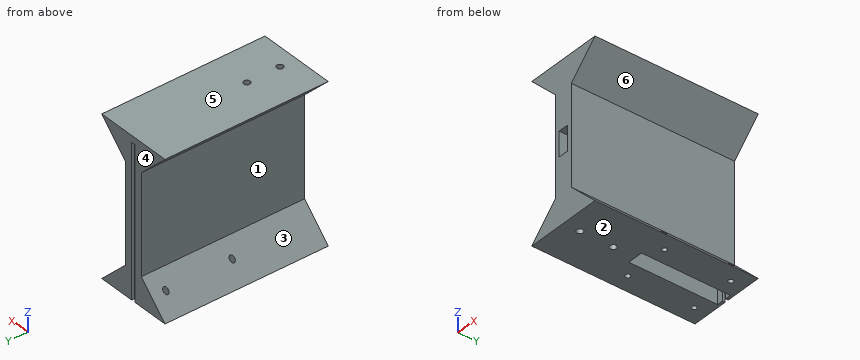
from build123d import *

# Parameters (mm, degrees)
BOSS_EXTRUDE1_DEPTH            = 125
SKETCH3_W                      = 12
SKETCH3_H                      = 68
CUT_EXTRUDE1_DEPTH             = 115.57
SKETCH4_W                      = 3.175
SKETCH4_H                      = 115.57
CUT_EXTRUDE2_DEPTH             = 3
CUT_EXTRUDE3_REACH             = 143.943
SKETCH5_W                      = 8
SKETCH5_H                      = 19.05
SKETCH6_R                      = 2.45745
CUT_EXTRUDE4_DEPTH             = 25.4
CUT_EXTRUDE5_START             = -25.4
SKETCH7_R                      = 2.45745
CUT_EXTRUDE5_DEPTH             = 25.4
TAP_DRILL_FOR_10_24_TAP1_D     = 3.7973
TAP_DRILL_FOR_10_24_TAP1_DEPTH = 30
TAP_DRILL_FOR_10_24_TAP1_TIP   = 1.140824014


with BuildPart() as part:
    # Sketch1 → Boss-Extrude1 (new body)
    with BuildSketch(Plane(origin=(0, 0, 0), x_dir=(1, 0, 0), z_dir=(0, 1, 0))):
        Polygon((-29.725, -60.325), (29.725, -60.325), (7.5, -38.1), (7.5, 38.1), (29.725, 60.325), (-29.725, 60.325), (-7.5, 38.1), (-7.5, -38.1), align=None)
    extrude(amount=BOSS_EXTRUDE1_DEPTH)

    # Sketch3 → Cut-Extrude1 (cut)
    with BuildSketch(Plane(origin=(0, 0, -60.325), x_dir=(-1, 0, 0), z_dir=(0, 0, -1))):
        with Locations((0, 89)):
            Rectangle(SKETCH3_W, SKETCH3_H)
    extrude(amount=-CUT_EXTRUDE1_DEPTH, mode=Mode.SUBTRACT)

    # Sketch4 → Cut-Extrude2 (cut)
    with BuildSketch(Plane(origin=(0, 125, 0), x_dir=(1, 0, 0), z_dir=(0, 1, 0))):
        with Locations((0, 2.54)):
            Rectangle(SKETCH4_W, SKETCH4_H)
    extrude(amount=-CUT_EXTRUDE2_DEPTH, mode=Mode.SUBTRACT)

    # Sketch5 → Cut-Extrude3 (cut, up to next)
    with BuildSketch(Plane.XZ, mode=Mode.PRIVATE) as cut_extrude3_sk1:
        Rectangle(SKETCH5_W, SKETCH5_H)
    cut_extrude3_tool1 = extrude(cut_extrude3_sk1.sketch, amount=-CUT_EXTRUDE3_REACH, mode=Mode.PRIVATE) & part.part
    add(cut_extrude3_tool1.solids().sort_by_distance((0, 0, 0))[0], mode=Mode.SUBTRACT)

    # Sketch6 → Cut-Extrude4 (cut)
    with BuildSketch(Plane(origin=(0, 0, -60.325), x_dir=(-1, 0, 0), z_dir=(0, 0, -1))):
        with Locations((0, 12.7)):
            Circle(SKETCH6_R)
        with Locations((0, 38.1)):
            Circle(SKETCH6_R)
    extrude(amount=-CUT_EXTRUDE4_DEPTH, mode=Mode.SUBTRACT)

    # Sketch7 → Cut-Extrude5 (cut)
    with BuildSketch(Plane.XY.offset(60.325).offset(CUT_EXTRUDE5_START)):
        with Locations(Location((0, 38.1, 0), (0, 0, 180))):
            Circle(SKETCH7_R)
        with Locations(Location((0, 12.7, 0), (0, 0, 180))):
            Circle(SKETCH7_R)
    extrude(amount=CUT_EXTRUDE5_DEPTH, mode=Mode.SUBTRACT)

    # Tap Drill for #10-24 Tap1
    with Locations(Plane(origin=(0, 0, -60.325), x_dir=(-1, 0, 0), z_dir=(0, 0, -1))):
        with Locations((-17.225, 114.15), (-17.225, 63.35), (17.225, 114.15), (17.225, 63.35)):
            Hole(TAP_DRILL_FOR_10_24_TAP1_D / 2, depth=TAP_DRILL_FOR_10_24_TAP1_DEPTH)
            with Locations((0, 0, -(TAP_DRILL_FOR_10_24_TAP1_DEPTH + TAP_DRILL_FOR_10_24_TAP1_TIP / 2))):  # 118° drill point
                Cone(0, TAP_DRILL_FOR_10_24_TAP1_D / 2, TAP_DRILL_FOR_10_24_TAP1_TIP, mode=Mode.SUBTRACT)


solid = part.part
Source: CAD feature listing. Evaluate the final solid. Frame: model axes, mm. Face numbers are marked on the shaded views. A direction names the side the tool comes from. Round coordinates to 2 decimals unless told otherwise and drop trailing zeros. Loops run counter-clockwise (first coordinate to the right, second up) from the corner with the lowest first, then second, coordinate; pieces in that order, holes last. Notation, with made-up numbers: (33, -34.5) - (70, -34.5) arc R13 cw to (70, -25.5) - close; hole circle Ø4 at (-16.5, 35). An arc over 180 degrees is marked (long way). Write item = value, one per line. Start each with the question number.
(1) Section query A-A, the plane x = 0. Output: boundary loops of the cut face in (y, z) (3 decimals), plus the area to 3 significant figures.
(2) Pin query (flat end, axial travel): pin 1 (1 mm diameter, centred on y = 91, z = 35, fed in from +X); pin 2 (4 mm diameter, centred on x = 0, y = 38.1, fed in from +Z) (3 decimals); pin 3 (10 mm diameter, centred on y = 19, z = -25.5, fed in from -X). Return the tip coordinate at first contact, or that it passes through.
(3) Section query C-C, the plane x = 17. Output: boundary loops of the cut face in (y, z) (3 decimals), plus the area to 3 significant figures.
(4) Section query D-D, the plane y = 96.5. Output: boundary loops of the cut face in (x, z) (3 decimals).
(5) Pull-direction query (Z, two-part tool) for the marked faces 1, 2, 3 and 4; classes: +Z half, -Z half, draft (parallel to the pull), parting line (faces both ways), or undercut.
(6) Section query B-B, the plane y = 12.7. Output: boundary loops of the cut face in (x, z) (3 decimals).
(7) Set-up query: the marked faces 5 and 6. Return all of +Z, -Z, +X, -X, +Y, -Y with unobstructed straight access to the full face (end or side cutting, diameter ignored); none if empty.
(8) Ray query, line 1 along Y through (x, z) = (0, -45); line 2 along Y through (x, z) = (-2, 27); line 3 along X through (y, z) = (64, 12). Return the intervals inside material, ascending. Write a range as from..to.
Conclusion:
q1.outline = (0, -60.325) - (10.243, -60.325) - (10.243, -34.925) - (15.157, -34.925) - (15.157, -60.325) - (35.643, -60.325) - (35.643, -34.925) - (40.557, -34.925) - (40.557, -60.325) - (55, -60.325) - (55, -9.525) - (0, -9.525) - close; (0, 9.525) - (55, 9.525) - (55, 55.245) - (125, 55.245) - (125, 60.325) - (40.557, 60.325) - (40.557, 34.925) - (35.643, 34.925) - (35.643, 60.325) - (15.157, 60.325) - (15.157, 34.925) - (10.243, 34.925) - (10.243, 60.325) - (0, 60.325) - close
q1.area = 5,440 mm2
q2.pin_1 = 7.5
q2.pin_2 = 34.925
q2.pin_3 = -7.5
q3.outline = (0, -60.325) - (61.465, -60.325) - (61.465, -47.6) - (0, -47.6) - close; (0, 47.6) - (125, 47.6) - (125, 60.325) - (0, 60.325) - close; (65.235, -60.325) - (112.265, -60.325) - (112.265, -47.6) - (65.235, -47.6) - close; (116.035, -60.325) - (125, -60.325) - (125, -47.6) - (116.035, -47.6) - close
q3.area = 3,090 mm2
q4.outline = (-29.725, -60.325) - (-6, -60.325) - (-6, 55.245) - (6, 55.245) - (6, -60.325) - (29.725, -60.325) - (7.5, -38.1) - (7.5, 38.1) - (29.725, 60.325) - (-29.725, 60.325) - (-7.5, 38.1) - (-7.5, -38.1) - close
q5.face_1 = undercut
q5.face_2 = -Z half
q5.face_3 = undercut
q5.face_4 = draft
q6.outline = (-29.725, -60.325) - (-2.457, -60.325) - (-2.457, -34.925) - (2.457, -34.925) - (2.457, -60.325) - (29.725, -60.325) - (7.5, -38.1) - (7.5, 38.1) - (29.725, 60.325) - (2.457, 60.325) - (2.457, 34.925) - (-2.457, 34.925) - (-2.457, 60.325) - (-29.725, 60.325) - (-7.5, 38.1) - (-7.5, -38.1) - close; hole (-4, -9.525) - (4, -9.525) - (4, 9.525) - (-4, 9.525) - close
q7.face_5 = +Z, +X, -X, +Y, -Y
q7.face_6 = +X, +Y, -Y
q8.line_1 = 0..10.24, 15.16..35.64, 40.56..55
q8.line_2 = 0..55, 123..125
q8.line_3 = -7.5..-6, 6..7.5
